Here's how the part is built. I have some questions about the finished solid (model axes, mm). A direction names the side the tool comes from. Give positions to 0.01 mm unless a question says otherwise; leave off trailing zeros. Write each loop counter-clockwise with the first axis right and the second up, starting at its lowest first coordinate (ties: lowest second). Pieces come first, ordered by that corner, then holes. Notation, with made-up numbers: (58, 45) -> (97, 45) arc R36 ccw to (97, 82) -> close; hole circle Ø7 at (57.5, -6). An arc over 180 degrees is marked (long way). Use one line per item in the form item = value.
```python
from build123d import *

# Parameters (mm, degrees)
F1_DEPTH = 10
F2_W     = 20
F2_H     = 30
F2_R     = 15
F3_DEPTH = 10.001
F4_R     = 4
F5_DEPTH = 15.4106812647


with BuildPart() as f1:
    # F0 (on Top) → F1 (new body)
    with BuildSketch(Plane.XY):
        Polygon((25, 86.6025403784), (-25, 86.6025403784), (-37.5, 64.9519052838), (-12.5, 21.6506350946), (12.5, 21.6506350946), (37.5, 64.9519052838), align=None)
    extrude(amount=F1_DEPTH)

    # F2 (on face) → F3 (cut, through all)
    with BuildSketch(Plane.XY.offset(10)):
        with Locations((0, 21.6506350946)):
            Rectangle(F2_W, F2_H)
        Polygon((-49.2403810568, 74.6169687933), (-23.2596189432, 59.6169687933), (-13.2596189432, 76.937476869), (-39.2403810568, 91.937476869), align=None)
        Polygon((39.2403810568, 91.937476869), (13.2596189432, 76.937476869), (23.2596189432, 59.6169687933), (49.2403810568, 74.6169687933), align=None)
        with Locations((0, 57.735026919)):
            Circle(F2_R)
    extrude(amount=-F3_DEPTH, mode=Mode.SUBTRACT)

    # F4 (on face) → F5 (cut, up to face)
    with BuildSketch(Plane(origin=(0, 0, 0), x_dir=(0.5, 0.8660254038, 0), z_dir=(0.8660254038, -0.5, 0))):
        with Locations((50, 5)):
            Circle(F4_R)
    extrude(amount=-F5_DEPTH, mode=Mode.SUBTRACT)


solid = f1.part
```
Q1. I want a section at C-C, the plane z = 6. Write out the boundary of the cut face in (x, y), and give its area (3 significant figures).
Result set:
outline = (-37.5, 64.95) -> (-12.5, 21.65) -> (-10, 21.65) -> (-10, 36.65) -> (10, 36.65) -> (10, 21.65) -> (12.5, 21.65) -> (23.06, 39.95) -> (10.61, 47.14) arc R15 cw (long way) to (14.49, 53.84) -> (26.94, 46.66) -> (37.5, 64.95) -> (36.25, 67.12) -> (23.26, 59.62) -> (13.26, 76.94) -> (26.25, 84.44) -> (25, 86.6) -> (-25, 86.6) -> (-26.25, 84.44) -> (-13.26, 76.94) -> (-23.26, 59.62) -> (-36.25, 67.12) -> close
area = 1,800 mm2
Q2. I want a section at A-A, the plane x = 0. Write out the boundary of the cut face in (y, z).
Result set:
outline = (36.65, 0) -> (42.74, 0) -> (42.74, 10) -> (36.65, 10) -> close; (72.74, 0) -> (86.6, 0) -> (86.6, 10) -> (72.74, 10) -> close
Q3. If we mould it in two halves opening along X, with no side actions, what happens to faces 1 (the face through (-11, 21.651, 5)), 2 (the face through (-25.616, 85.535, 4.93)), 3 (the face through (25.634, 85.505, 4.93)), 4 (the face through (16.849, 43.393, 5.176))? For each: +X half, -X half, draft (parallel to the pull), parting line (faces both ways), or undercut.
Result set:
face_1 = draft
face_2 = -X half
face_3 = +X half
face_4 = undercut
Q4. Which directions (+Z, -Z, +X, -X, +Y, -Y) give clear straight access to the entire face, cutting with the end or side of a thin tool? Please do faces 5 (the face through (18.19, 68.4, 5.07)), 6 (the face through (-25.175, 43.604, 4.93)), 7 (the face through (-19.664, 80.635, 5.07)), 8 (the face through (10, 29, 5)).
Result set:
face_5 = +Z, -Z
face_6 = +Z, -Z, -X, -Y
face_7 = +Z, -Z, -X
face_8 = +Z, -Z, -Y
Q5. If I drill on line 1 along Y through (x, z) = (0, 5.5); line 2 along X through (y, z) = (62.5, 3.75); line 3 along Y through (x, z) = (23, 8.5), over which ranges is the centre line in solid material (lowest first)? Write a range as from..to.
Result set:
line_1 = 36.65..42.74, 72.74..86.6
line_2 = -36.08..-28.25, -21.6..-14.22, 14.22..21.6, 28.25..36.08
line_3 = 39.84..42.22, 46.69..60.07, 82.56..86.6
Q6. Will these pins go through, and if not, where does the flat tip stop? pin 1 Ø8 at (x, y) = (29, 56.5) entering from -Z; pin 2 Ø4 at (y, z) = (57.5, 5) entering from -X; pin 3 Ø5 at (y, z) = (31, 6) entering from -X; pin 4 Ø3 at (x, z) = (3, 3.5) entering from -Y.
Result set:
pin_1 = 0
pin_2 = -34.35
pin_3 = -19.34
pin_4 = 36.65
Q7. I want a section at D-D, the plane x = 16. Count the separate pieces of the cut face and the enclosed holes in it, and give its area (3 significant figures).
Result set:
separate_pieces = 2
enclosed_holes = 1
area = 468 mm2
Q8. I want a section at B-B, the plane y = 55.5. Write out the boundary of the cut face in (x, z).
Result set:
outline = (-32.04, 0) -> (-14.83, 0) -> (-14.83, 10) -> (-32.04, 10) -> close; (14.83, 0) -> (32.04, 0) -> (32.04, 10) -> (14.83, 10) -> close
